Can you work these out from the drawing? Everything is in mm from the part's minimum corner. A direction names the side the tool comes from. Coordinates: 2 decimals unless noted, no trailing zeros. Order: outer loops, then holes, each group sorted by start corner. A loop starts at its lowest first (then second) coordinate and runs counter-clockwise, first axis right, second up. Notation, with made-up numbers: (3, 89) - (59, 89) arc R19 ccw to (59, 93) - close; hole circle Ø5 at (35.25, 63). An arc over 180 degrees is marked (long way). Use a Markdown table: item, result. Add a question column.
(1) On a 3-axis mill with a long thin cutter (end or side, diameter ignored), from which of +Z, -Z, +X, -X, +Y, -Y can I reach the whole of each face in a straight line? I mean the marked faces 1 and 2. Say none if no direction works.
(2) I want a section at C-C (y = 105). List the corners of the cut face in (x, z) for me, and give its area (3 significant figures).
(3) If I drill on L1, parallel to Y at x = 100, z = 2; L2, parallel to Y at x = 580, z = 437; L3, parallel to X at y = 236, z = 92, over which ranges is the centre line in solid material (lowest first)? Write a range as [from, to].
(4) For pin 1 Ø20 at (x, y) = (579.5, 48) entering from +Z; pin 2 Ø25 at (x, y) = (812, 334.5) entering from -Z, each with a flat end and sliding along its axis, tell me the tip position at first contact or that it passes through.
(5) I want a section at D-D (x = 445). List the corners of the cut face in (y, z) for me.
(6) I want a section at A-A (x = 340). List the corners of the cut face in (y, z) for me, and give its area (3 significant figures).
(7) I want a section at B-B (z = 99). List the corners of the cut face in (x, y) for me.
(8) We'd pull the mould along Z, two halves only. Please class the marked faces 3, 4 and 5: pulls with the +Z half, pulls with the -Z half, needs draft (parallel to the pull), parting line crosses it, or undercut.
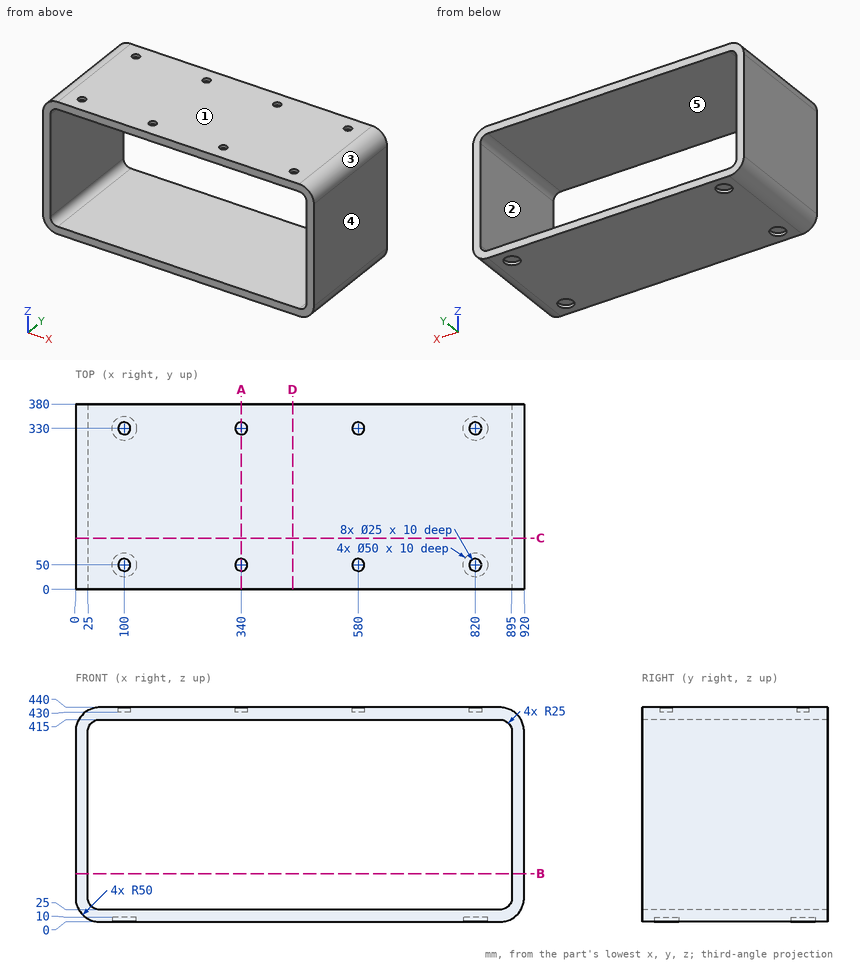
Answers follow:
| question | item | result |
|---|---|---|
| 1 | face 1 | +Z, +X, -X, +Y, -Y |
| 1 | face 2 | +Y, -Y |
| 2 | outline | (0, 50) arc R50 ccw to (50, 0) - (870, 0) arc R50 ccw to (920, 50) - (920, 390) arc R50 ccw to (870, 440) - (50, 440) arc R50 ccw to (0, 390) - close; hole (25, 50) arc R25 ccw to (50, 25) - (870, 25) arc R25 ccw to (895, 50) - (895, 390) arc R25 ccw to (870, 415) - (50, 415) arc R25 ccw to (25, 390) - close |
| 2 | area | 63,900 mm² |
| 3 | L1 | y = [0, 25], [75, 305], [355, 380] |
| 3 | L2 | y = [0, 37.5], [62.5, 317.5], [342.5, 380] |
| 3 | L3 | x = [0, 25], [895, 920] |
| 4 | pin 1 | stops at z = 430 |
| 4 | pin 2 | stops at z = 10 |
| 5 | outline | (0, 0) - (380, 0) - (380, 25) - (0, 25) - close; (0, 415) - (380, 415) - (380, 440) - (0, 440) - close |
| 6 | outline | (0, 0) - (380, 0) - (380, 25) - (0, 25) - close; (0, 415) - (380, 415) - (380, 440) - (342.5, 440) - (342.5, 430) - (317.5, 430) - (317.5, 440) - (62.5, 440) - (62.5, 430) - (37.5, 430) - (37.5, 440) - (0, 440) - close |
| 6 | area | 18,500 mm² |
| 7 | outline | (0, 0) - (25, 0) - (25, 380) - (0, 380) - close; (895, 0) - (920, 0) - (920, 380) - (895, 380) - close |
| 8 | face 3 | pulls with the +Z half |
| 8 | face 4 | needs draft |
| 8 | face 5 | undercut |
